Could you check a few things on this model? Use its own coordinates, in mm. A direction names the side the tool comes from. Give positions to 0.01 mm unless a question says otherwise; leave off trailing zeros. Order: outer loops, then holes, each group sorted by start corner. A loop starts at its lowest first (then second) coordinate and runs counter-clockwise, first axis right, second up. Notation, with made-up numbers: (-26.5, 23) -> (28.5, 23) arc R22 ccw to (28.5, 62) -> close; hole circle Ø6 at (-16, -4). An arc over 180 degrees is marked (long way). Answer as CSV lines item,"result". Start each with the question number.
(1) I need wall thicknesses on L1, parallel to Z at x = 0, y = -62.5; L2, parallel to Z at x = 0, y = -164; L3, parallel to X at y = -107, z = 15. Which ranges of each line are inside material? Lowest first, please.
(2) On a 3-axis mill with a long thin cutter (end or side, diameter ignored), from which of +Z, -Z, +X, -X, +Y, -Y can I reach the whole of each face in a straight line? I mean faces 1 (the face through (-63.5, -63, -1)), 2 (the face through (27, -127, 29)). Say none if no direction works.
(3) Will this pin go through, and if not, where does the flat tip stop? pin 1 Ø2 at (x, z) = (-32.5, -24.5) entering from -Y.
(4) I want a section at D-D (x = -43.5). Please give me the cut outline in (y, z).
(5) I want a section at C-C (y = -60). Please give me the cut outline in (x, z).
(6) I want a section at B-B (z = 0). Please give me the cut outline in (x, y), plus the area to 3 significant figures.
(7) I want a section at A-A (x = 0). Please give me the cut outline in (y, z), plus the area to 3 significant figures.
```python
from build123d import *

# Parameters (mm, degrees)
F0_W     = 127
F0_H     = 127
F1_DEPTH = 127
F2_R     = 31.75
F3_DEPTH = 127.001
F4_R     = 38.1
F4_R_2   = 31.75
F5_DEPTH = 76.2


with BuildPart() as f1:
    # F0 (on Front) → F1 (new body)
    with BuildSketch(Plane.XZ):
        Rectangle(F0_W, F0_H)
    extrude(amount=F1_DEPTH)

    # F2 (on face) → F3 (cut, through all)
    with BuildSketch(Plane.XZ.offset(127)):
        Circle(F2_R)
    extrude(amount=-F3_DEPTH, mode=Mode.SUBTRACT)

    # F4 (on face) → F5 (join)
    with BuildSketch(Plane.XZ.offset(127)):
        Circle(F4_R)
        Circle(F4_R_2, mode=Mode.SUBTRACT)
    extrude(amount=F5_DEPTH)


solid = f1.part
```
Final values:
1,L1,"-63.5 to -31.75, 31.75 to 63.5"
1,L2,"-38.1 to -31.75, 31.75 to 38.1"
1,L3,"-63.5 to -27.98, 27.98 to 63.5"
2,face 1,"+Z, -Z, -X, +Y, -Y"
2,face 2,"-Y"
3,pin 1,"y = -127"
4,outline,"(-127, -63.5) -> (0, -63.5) -> (0, 63.5) -> (-127, 63.5) -> close"
5,outline,"(-63.5, -63.5) -> (63.5, -63.5) -> (63.5, 63.5) -> (-63.5, 63.5) -> close; hole circle Ø63.5 at (0, 0)"
6,outline,"(-63.5, -127) -> (-38.1, -127) -> (-38.1, -203.2) -> (-31.75, -203.2) -> (-31.75, 0) -> (-63.5, 0) -> close; (31.75, -203.2) -> (38.1, -203.2) -> (38.1, -127) -> (63.5, -127) -> (63.5, 0) -> (31.75, 0) -> close"
6,area,"9,030 mm²"
7,outline,"(-203.2, -38.1) -> (-127, -38.1) -> (-127, -63.5) -> (0, -63.5) -> (0, -31.75) -> (-203.2, -31.75) -> close; (-203.2, 31.75) -> (0, 31.75) -> (0, 63.5) -> (-127, 63.5) -> (-127, 38.1) -> (-203.2, 38.1) -> close"
7,area,"9,030 mm²"
